The model under review builds one solid part; all positions refer to its coordinate system, in mm. Face numbers are marked on the shaded views. A direction names the side the tool comes from. Coordinates: 2 decimals unless noted, no trailing zeros. Order: outer loops, then holes, each group sorted by start corner. A loop starts at its lowest first (then second) coordinate and runs counter-clockwise, first axis right, second up. Notation, with made-up numbers: (47, 39.5) - (83, 39.5) arc R14 ccw to (83, 50.5) - close; hole circle Ø2 at (31.25, -26). An arc over 180 degrees is marked (long way). Answer in a Markdown table with one row per item.
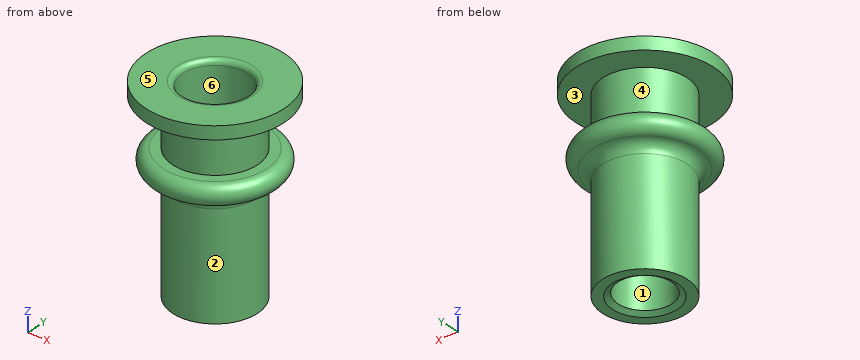
```python
from build123d import *


with BuildPart() as part:
    # Sketch1 → Revolve1 (revolve)
    with BuildSketch(Plane(origin=(0, 0, 0), x_dir=(0, 0, -1), z_dir=(1, 0, 0)), mode=Mode.PRIVATE) as revolve1_sk:
        with BuildLine():
            Line((0, 2.8067), (0, 5.1562))
            Line((0, 5.1562), (0.9652, 5.1562))
            Line((0.9652, 5.1562), (0.9652, 3.175))
            Line((0.9652, 3.175), (4.572, 3.175))
            Line((4.572, 3.175), (4.572, 3.8862))
            ThreePointArc((4.572, 3.8862), (5.334, 4.6482), (6.096, 3.8862))
            Line((6.096, 3.8862), (6.096, 3.937))
            ThreePointArc((6.096, 3.937), (6.319184633, 3.398184633), (6.858, 3.175))
            Line((6.858, 3.175), (14.732, 3.175))
            Line((14.732, 3.175), (14.732, 2.4257))
            Line((14.732, 2.4257), (14.497364851, 2.0193))
            Line((14.497364851, 2.0193), (7.092635149, 2.0193))
            Line((7.092635149, 2.0193), (6.858, 2.4257))
            Line((6.858, 2.4257), (0.381, 2.4257))
            ThreePointArc((0.381, 2.4257), (0.111592316, 2.537292316), (0, 2.8067))
        make_face()
    revolve(revolve1_sk.sketch.rotate(Axis((0, 0, 2.825013871), (0, 0, 1)), 90), axis=Axis((0, 0, 2.825013871), (0, 0, 1)))


solid = part.part
```
Item 1: Tool access review of the marked faces 1, 2 and 3: name each direction out of +Z, -Z, +X, -X, +Y, -Y from which nothing blocks a thin tool from reaching the whole face with its end or side.
Check values:
| item | result |
|---|---|
| face 1 | +Z, -Z |
| face 2 | -Z |
| face 3 | none |
Item 2: We need section C-C, the plane z = -9. Write out the cut boundary in (x, y) (3 decimals).
Check values:
| item | result |
|---|---|
| outline | circle Ø6.35 at (0, 0); hole circle Ø4.039 at (0, 0) |
Item 3: Clearance check with flat-ended pins moving along their axes: pin 1 Ø5 at (y, z) = (-1, -12.5) entering from +X (3 decimals); pin 2 Ø1 at (x, y) = (-1, 1.5) entering from -Z; pin 3 Ø3 at (x, z) = (2.5, -5.5) entering from -Y. State where each tip first meets the part, or that it passes through.
Check values:
| item | result |
|---|---|
| pin 1 | x = 3.175 |
| pin 2 | z = -14.66 |
| pin 3 | y = -4.54 |
Item 4: Mouldability with a two-part tool opening along X and no side actions: class the marked faces 4, 5 and 6 as +X half, -X half, draft (parallel to the pull), parting line (faces both ways), or undercut.
Check values:
| item | result |
|---|---|
| face 4 | parting line |
| face 5 | draft |
| face 6 | undercut |
Item 5: To check wall thickness, follow line 1 (Y direction, x = 0, z = -3.5) (3 decimals); line 2 (Y direction, x = 0, z = -11) (3 decimals); line 3 (X direction, y = 0.75, z = -13.25). State the ranges of each line that lie inside material, in increasing order. Write a range as from..to.
Check values:
| item | result |
|---|---|
| line 1 | -3.175..-2.426, 2.426..3.175 |
| line 2 | -3.175..-2.019, 2.019..3.175 |
| line 3 | -3.09..-1.87, 1.87..3.09 |
Item 6: We need section D-D, the plane z = -4. Write out the cut boundary in (x, y) (3 decimals).
Check values:
| item | result |
|---|---|
| outline | circle Ø6.35 at (0, 0); hole circle Ø4.851 at (0, 0) |
